Here's how the part is built. I have some questions about the finished solid (model axes, mm). Face numbers are marked on the shaded views. Give positions to 0.01 mm unless a question says otherwise; leave off trailing zeros. Write each loop counter-clockwise with the first axis right and the second up, starting at its lowest first coordinate (ties: lowest second). Pieces come first, ordered by that corner, then holes. Notation, with made-up numbers: (70.5, 86) -> (100.5, 86) arc R7 ccw to (100.5, 94) -> close; hole circle Ø4 at (23.5, 43). An arc over 180 degrees is marked (long way). Return JSON: item names as keys, results as strings.
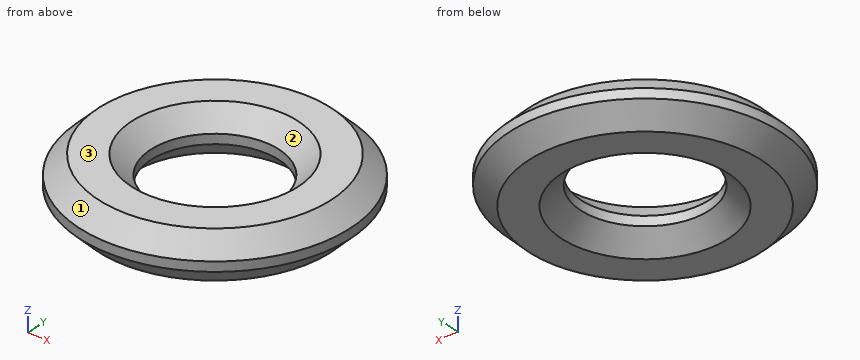
from build123d import *

# Parameters (mm, degrees)
ESBO_O1_R                = 5.7
ESBO_O1_R_2              = 2.7
RESSALTO_EXTRUS_O1_DEPTH = 2
CHANFRO1_SIZE            = 0.8


with BuildPart() as part:
    # Esboço1 → Ressalto-extrusão1 (new body)
    with BuildSketch(Plane.XY):
        Circle(ESBO_O1_R)
        Circle(ESBO_O1_R_2, mode=Mode.SUBTRACT)
    extrude(amount=RESSALTO_EXTRUS_O1_DEPTH)

    # Chanfro1
    chanfro1_edges = [part.edges().sort_by_distance(p)[0] for p in [
        (-5.7, 0, 0),
        (-5.7, 0, 2),
        (-2.7, 0, 0),
        (-2.7, 0, 2),
    ]]
    chamfer(chanfro1_edges, length=CHANFRO1_SIZE)


solid = part.part
1. Suppose I cut it at D-D, the plane z = 1.65. List the corners of the cut face in (x, y) for me, and give its area (3 significant figures).
Taken from the geometry:
{"outline": "circle Ø10.5 at (0, 0); hole circle Ø6.3 at (0, 0)", "area": "55.4 mm²"}
2. Suppose I cut it at C-C, the plane z = 0.65. List the corners of the cut face in (x, y) for me, and give its area (3 significant figures).
Taken from the geometry:
{"outline": "circle Ø11.1 at (0, 0); hole circle Ø5.7 at (0, 0)", "area": "71.3 mm²"}
3. If I drill on line 1 (Y direction, x = 0, z = 1.1); line 2 (Y direction, x = -2, z = 1.3); line 3 (X direction, y = 0.25, z = 1.4), over which ranges is the centre line in solid material (lowest first)? Write a range as [from, to].
Taken from the geometry:
{"line 1": "y = [-5.7, -2.7], [2.7, 5.7]", "line 2": "y = [-5.23, -1.96], [1.96, 5.23]", "line 3": "x = [-5.49, -2.89], [2.89, 5.49]"}
4. For pin 1 Ø1 at (x, y) = (-1.5, -1) entering from +Z, with a flat end and sliding along its axis, tell me the tip position at first contact or that it passes through.
Taken from the geometry:
{"pin 1": "passes through"}
5. If we mould it in two halves opening along X, with no side actions, what happens to the marked faces 1, 2 and 3? For each: released by +X, released by -X, zero draft, split by the parting line, or undercut.
Taken from the geometry:
{"face 1": "split by the parting line", "face 2": "undercut", "face 3": "zero draft"}
6. Suppose I cut it at A-A, the plane x = 0. List the corners of the cut face in (y, z) for me, and give its area (3 significant figures).
Taken from the geometry:
{"outline": "(-5.7, 0.8) -> (-4.9, 0) -> (-3.5, 0) -> (-2.7, 0.8) -> (-2.7, 1.2) -> (-3.5, 2) -> (-4.9, 2) -> (-5.7, 1.2) -> close; (2.7, 0.8) -> (3.5, 0) -> (4.9, 0) -> (5.7, 0.8) -> (5.7, 1.2) -> (4.9, 2) -> (3.5, 2) -> (2.7, 1.2) -> close", "area": "9.44 mm²"}
